```python
from build123d import *

# Parameters (mm, degrees)
SKETCH1_W           = 56
SKETCH1_H           = 32
SKETCH1_W_2         = 50
SKETCH1_H_2         = 26
BOSS_EXTRUDE1_DEPTH = 3
SKETCH2_W           = 3
SKETCH2_H           = 3
BOSS_EXTRUDE2_DEPTH = 40
BOSS_EXTRUDE3_DEPTH = 3
BOSS_EXTRUDE4_DEPTH = 3
SKETCH5_W           = 3
SKETCH5_H           = 26
BOSS_EXTRUDE5_DEPTH = 3
SKETCH6_W           = 50
SKETCH6_H           = 3
SKETCH6_W_2         = 3
BOSS_EXTRUDE7_DEPTH = 3
SKETCH7_W           = 3
SKETCH7_H           = 3
BOSS_EXTRUDE8_DEPTH = 15
SKETCH8_W           = 3
SKETCH8_H           = 26
SKETCH8_W_2         = 6
SKETCH8_H_2         = 3
BOSS_EXTRUDE9_DEPTH = 3


with BuildPart() as part:
    # Sketch1 → Boss-Extrude1 (new body)
    with BuildSketch(Plane(origin=(0, 0, 0), x_dir=(1, 0, 0), z_dir=(0, 1, 0))):
        Rectangle(SKETCH1_W, SKETCH1_H)
        Rectangle(SKETCH1_W_2, SKETCH1_H_2, mode=Mode.SUBTRACT)
    extrude(amount=BOSS_EXTRUDE1_DEPTH)

    # Sketch2 → Boss-Extrude2 (add)
    with BuildSketch(Plane(origin=(0, 0, 0), x_dir=(1, 0, 0), z_dir=(0, 1, 0))):
        with Locations((26.5, 14.5)):
            Rectangle(SKETCH2_W, SKETCH2_H)
        with Locations((26.5, -14.5)):
            Rectangle(SKETCH2_W, SKETCH2_H)
        with Locations((-26.5, -14.5)):
            Rectangle(SKETCH2_W, SKETCH2_H)
        with Locations((-26.5, 14.5)):
            Rectangle(SKETCH2_W, SKETCH2_H)
    extrude(amount=BOSS_EXTRUDE2_DEPTH)

    # Sketch3 → Boss-Extrude3 (add)
    with BuildSketch(Plane.XY.offset(16)):
        Polygon((28, 10), (28, 5), (29.7, 5), (29.7, 8.2), (32.9, 8.2), (32.9, 6.6), (36.1, 6.6), (36.1, 5), (38, 5), (38, 10), align=None)
        Polygon((28, 5), (28, 0), (38, 0), (38, 5), (36.1, 5), (36.1, 3.4), (32.9, 3.4), (32.9, 1.8), (29.7, 1.8), (29.7, 5), align=None)
    boss_extrude3 = extrude(amount=-BOSS_EXTRUDE3_DEPTH)

    # Mirror1: Boss-Extrude3 across plane
    add(boss_extrude3.mirror(Plane.XY))

    # Sketch4 → Boss-Extrude4 (add)
    with BuildSketch(Plane.XY.offset(16)):
        Polygon((5, 0), (0, 0), (-5, 0), (-5, -10), (0, -10), (5, -10), align=None)
        Polygon((1.6, -8.1), (0, -8.1), (-1.6, -8.1), (-1.6, -4.9), (-3.2, -4.9), (-3.2, -1.7), (3.2, -1.7), (3.2, -4.9), (1.6, -4.9), align=None, mode=Mode.SUBTRACT)
    boss_extrude4 = extrude(amount=-BOSS_EXTRUDE4_DEPTH)

    # Mirror2: Boss-Extrude4 across plane
    add(boss_extrude4.mirror(Plane.XY))

    # Sketch5 → Boss-Extrude5 (add)
    with BuildSketch(Plane(origin=(0, 3, 0), x_dir=(1, 0, 0), z_dir=(0, 1, 0))):
        with Locations((-17, 0)):
            Rectangle(SKETCH5_W, SKETCH5_H)
        with Locations((-8, 0)):
            Rectangle(SKETCH5_W, SKETCH5_H)
        with Locations((8, 0)):
            Rectangle(SKETCH5_W, SKETCH5_H)
        with Locations((17, 0)):
            Rectangle(SKETCH5_W, SKETCH5_H)
    extrude(amount=-BOSS_EXTRUDE5_DEPTH)

    # Sketch6 → Boss-Extrude7 (add)
    # profile 1 of 4: a face of its own
    with BuildSketch(Plane(origin=(0, 40, 0), x_dir=(1, 0, 0), z_dir=(0, 1, 0))):
        Polygon((-28, -16), (25, -16), (25, -13), (28, -13), (28, 16), (-28, 16), align=None)
        Polygon((25, -9), (25, -13), (-25, -13), (-25, -9), (-25, -6), (-25, 6), (-25, 9), (-25, 13), (25, 13), (25, 9), (25, 6), (25, -6), align=None, mode=Mode.SUBTRACT)
    # profile 2 of 4: a face of its own
    with BuildSketch(Plane(origin=(0, 40, 0), x_dir=(1, 0, 0), z_dir=(0, 1, 0))):
        with Locations((0, -7.5)):
            Rectangle(SKETCH6_W, SKETCH6_H)
    # profile 3 of 4: a face of its own
    with BuildSketch(Plane(origin=(0, 40, 0), x_dir=(1, 0, 0), z_dir=(0, 1, 0))):
        with Locations((0, 7.5)):
            Rectangle(SKETCH6_W, SKETCH6_H)
    # profile 4 of 4: a face of its own
    with BuildSketch(Plane(origin=(0, 40, 0), x_dir=(1, 0, 0), z_dir=(0, 1, 0))):
        with Locations((26.5, -14.5)):
            Rectangle(SKETCH6_W_2, SKETCH6_H)
    extrude(amount=BOSS_EXTRUDE7_DEPTH)

    # Sketch7 → Boss-Extrude8 (add)
    with BuildSketch(Plane(origin=(0, 43, 0), x_dir=(1, 0, 0), z_dir=(0, 1, 0))):
        with Locations((-26.5, -14.5)):
            Rectangle(SKETCH7_W, SKETCH7_H)
        with Locations((-26.5, 14.5)):
            Rectangle(SKETCH7_W, SKETCH7_H)
        with Locations((26.5, 14.5)):
            Rectangle(SKETCH7_W, SKETCH7_H)
        with Locations((26.5, -14.5)):
            Rectangle(SKETCH7_W, SKETCH7_H)
    extrude(amount=BOSS_EXTRUDE8_DEPTH)

    # Sketch8 → Boss-Extrude9 (add)
    # profile 1 of 5: a face of its own
    with BuildSketch(Plane(origin=(0, 58, 0), x_dir=(1, 0, 0), z_dir=(0, 1, 0))):
        Polygon((-25, 16), (-25, 13), (-28, 13), (-28, -16), (28, -16), (28, 16), align=None)
        Polygon((25, 13), (25, -13), (15.5, -13), (12.5, -13), (9.5, -13), (0, -13), (-9.5, -13), (-15.5, -13), (-25, -13), (-25, 13), (-15.5, 13), (-9.5, 13), (9.5, 13), (12.5, 13), (15.5, 13), align=None, mode=Mode.SUBTRACT)
    # profile 2 of 5: a face of its own
    with BuildSketch(Plane(origin=(0, 58, 0), x_dir=(1, 0, 0), z_dir=(0, 1, 0))):
        with Locations((11, 0)):
            Rectangle(SKETCH8_W, SKETCH8_H)
    # profile 3 of 5: a face of its own
    with BuildSketch(Plane(origin=(0, 58, 0), x_dir=(1, 0, 0), z_dir=(0, 1, 0))):
        with Locations((14, 0)):
            Rectangle(SKETCH8_W, SKETCH8_H)
    # profile 4 of 5: a face of its own
    with BuildSketch(Plane(origin=(0, 58, 0), x_dir=(1, 0, 0), z_dir=(0, 1, 0))):
        with Locations((-12.5, 0)):
            Rectangle(SKETCH8_W_2, SKETCH8_H)
    # profile 5 of 5: a face of its own
    with BuildSketch(Plane(origin=(0, 58, 0), x_dir=(1, 0, 0), z_dir=(0, 1, 0))):
        with Locations((-26.5, 14.5)):
            Rectangle(SKETCH8_W, SKETCH8_H_2)
    extrude(amount=BOSS_EXTRUDE9_DEPTH)


solid = part.part
```
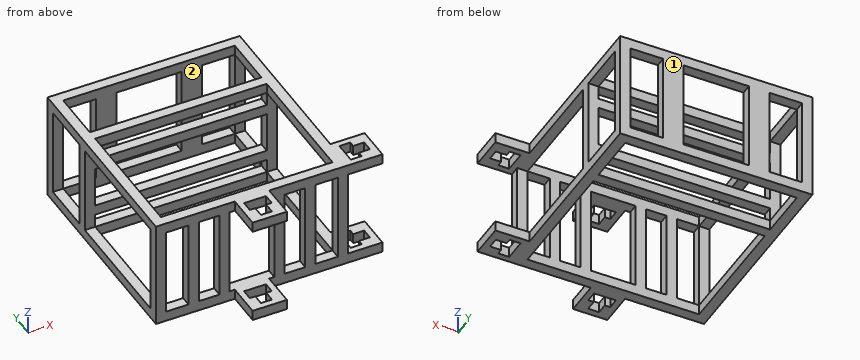
Input: part model. Units: mm. Frame: model coordinates. Face numbers are marked on the shaded views. Coordinates: 2 decimals unless noted, no trailing zeros. Loops run counter-clockwise (first coordinate to the right, second up) from the corner with the lowest first, then second, coordinate; pieces in that order, holes last. Notation, with made-up numbers: M 85,13 L 117,13 A12 ccw 117,19 Z; hole C 55,-28 d2. An arc over 180 degrees is marked long. Use a Markdown table: item, result. Add a question column.
1) Pin query (flat end, axial travel): P1, Ø8, axis at y = 40.5, z = 12.5, coming from the +X side; P2, Ø3.5, axis at x = -26, z = 5, coming from the -Y side; P3, Ø0.9, axis at x = 30.5, z = 14, coming from the +Y side. Return the tip coordinate at first contact, or that it passes through.
2) Section B-B, the plane y = 37. Return the cut outline in (x, z), plus the area to 3 significant figures.
3) Line query: L1, parallel to Y at x = -13, z = 13.5; L2, parallel to X at y = 2.5, z = 6; L3, parallel to Z at x = -20.5, y = 2.5. Output: solid intervals per line, ascending. Write a range as from..to.
4) Section A-A, the plane x = -14. Return the cut outline in (y, z), plus the area to 3 significant figures.
5) Section C-C, the plane x = 24. Give the number of separate pieces and of enclosed holes in the cut face, plus the area to 3 significant figures.
6) Draft query along Y for the marked faces 1 and 2. Return one class per face: +Y half, -Y half, draft (parallel to the pull), parting line (faces both ways), or undercut.
Answer below:
| question | item | result |
|---|---|---|
| 1 | P1 | x = 28 |
| 1 | P2 | y = 0 |
| 1 | P3 | y = 10 |
| 2 | outline | M -28,-16 L -25,-16 L -25,-13 L -28,-13 Z; M -28,13 L -25,13 L -25,16 L -28,16 Z; M 25,-16 L 28,-16 L 28,-13 L 25,-13 Z; M 25,13 L 28,13 L 28,16 L 25,16 Z |
| 2 | area | 36.0 mm2 |
| 3 | L1 | 0..3, 40..43, 58..61 |
| 3 | L2 | -28..-25, -18.5..-15.5, -9.5..-6.5, 6.5..9.5, 15.5..18.5, 25..28 |
| 3 | L3 | -16..-13, 13..16 |
| 4 | outline | M 0,-16 L 3,-16 L 3,-13 L 0,-13 Z; M 0,13 L 3,13 L 3,16 L 0,16 Z; M 40,-16 L 43,-16 L 43,-13 L 40,-13 Z; M 40,-9 L 43,-9 L 43,-6 L 40,-6 Z; M 40,6 L 43,6 L 43,9 L 40,9 Z; M 40,13 L 43,13 L 43,16 L 40,16 Z; M 58,-16 L 61,-16 L 61,16 L 58,16 Z |
| 4 | area | 150 mm2 |
| 5 | separate pieces | 8 |
| 5 | enclosed holes | 0 |
| 5 | area | 72.0 mm2 |
| 6 | face 1 | +Y half |
| 6 | face 2 | undercut |
